The listing builds one solid part. Answer for the finished solid, in the listing's coordinates (mm). A direction names the side the tool comes from. Round coordinates to 2 decimals unless told otherwise and drop trailing zeros. Loops run counter-clockwise (first coordinate to the right, second up) from the corner with the lowest first, then second, coordinate; pieces in that order, holes last. Notation, with made-up numbers: M 8.5,-38 L 43.5,-38 A10 ccw 43.5,-20 Z; hole C 34.5,64 d11. An arc over 180 degrees is marked long. Answer as a JSON object with one key per item and string values.
```python
from build123d import *

# Parameters (mm, degrees)
F1_DEPTH = 20
F2_R     = 2
F3_R     = 3.25
F4_DEPTH = 50
F5_R     = 3.25
F6_DEPTH = 25


with BuildPart() as f1:
    # F0 (on Top) → F1 (new body)
    with BuildSketch(Plane.XY):
        with BuildLine():
            Line((0, 32), (0, 0))
            Line((0, 0), (1.5, 0))
            Line((1.5, 0), (1.5, 32))
            ThreePointArc((1.5, 32), (1.93934, 33.06066), (3, 33.5))
            Line((3, 33.5), (15, 33.5))
            ThreePointArc((15, 33.5), (17.12132, 34.37868), (18, 36.5))
            Line((18, 36.5), (18, 50))
            Line((18, 50), (16.5, 50))
            Line((16.5, 50), (16.5, 36.5))
            ThreePointArc((16.5, 36.5), (16.06066, 35.43934), (15, 35))
            Line((15, 35), (3, 35))
            ThreePointArc((3, 35), (0.87868, 34.12132), (0, 32))
        make_face()
    extrude(amount=F1_DEPTH)

    # F2
    f2_edges = [f1.edges().sort_by_distance(p)[0] for p in [
        (0.75, 0, 20),
        (0.75, 0, 0),
        (17.25, 50, 20),
        (17.25, 50, 0),
    ]]
    fillet(f2_edges, radius=F2_R)

    # F3 (on face) → F4 (cut)
    with BuildSketch(Plane.YZ.offset(18)):
        with Locations((9, 10)):
            Circle(F3_R)
    extrude(amount=-F4_DEPTH, mode=Mode.SUBTRACT)

    # F5 (on face) → F6 (cut)
    with BuildSketch(Plane.XZ.offset(-33.5)):
        with Locations((9, 10)):
            Circle(F5_R)
    extrude(amount=-F6_DEPTH, mode=Mode.SUBTRACT)


solid = f1.part
```
Item 1: The part is cut by section B-B (z = 10). Give the vertices of the cut face in (x, y).
Values follow:
{"outline": "M 0,0 L 1.5,0 L 1.5,5.75 L 0,5.75 Z; M 0,12.25 L 1.5,12.25 L 1.5,32 A1.5 cw 3,33.5 L 5.75,33.5 L 5.75,35 L 3,35 A3 ccw 0,32 Z; M 12.25,33.5 L 15,33.5 A3 ccw 18,36.5 L 18,50 L 16.5,50 L 16.5,36.5 A1.5 cw 15,35 L 12.25,35 Z"}
Item 2: Straight lines are drawn through the part: line 1 (Z direction, x = 0.4, y = 9); line 2 (Y direction, x = 7, z = 19); line 3 (X direction, y = 18, z = 1.5). For each, find the intervals that lie inside material, in ascending order.
Values follow:
{"line 1": "0 to 6.75, 13.25 to 20", "line 2": "33.5 to 35", "line 3": "0 to 1.5"}
Item 3: Flat-ended cylindrical pins translate along their axes: P1, Ø6, axis at y = 19, z = 8, coming from the +X side; P2, Ø2, axis at x = 15, z = 10, coming from the -Y side; P3, Ø6, axis at x = 6, z = 13.5, coming from the +Y side. Find the tip coordinate at first contact, or state that the pin passes through.
Values follow:
{"P1": "x = 1.5", "P2": "y = 33.5", "P3": "y = 35"}
Item 4: The part is cut by section C-C (y = 9). Give the vertices of the cut face in (x, z), then the cut area to 4 significant figures.
Values follow:
{"outline": "M 0,0 L 1.5,0 L 1.5,6.75 L 0,6.75 Z; M 0,13.25 L 1.5,13.25 L 1.5,20 L 0,20 Z", "area": "20.25 mm^2"}
Item 5: Determine the mould class of faces 4 (the face through (0.76, 0.57, 0.6)), 5 (the face through (16.5, 43, 10)), 6 (the face through (5.753, 34.24, 10.143)) for opening direction Z: released by +Z, released by -Z, zero draft, split by the parting line, or undercut.
Values follow:
{"face 4": "released by -Z", "face 5": "zero draft", "face 6": "undercut"}
Item 6: The part is cut by section A-A (x = 9). Give the vertices of the cut face in (y, z), then the cut area to 4 significant figures.
Values follow:
{"outline": "M 33.5,0 L 35,0 L 35,6.75 L 33.5,6.75 Z; M 33.5,13.25 L 35,13.25 L 35,20 L 33.5,20 Z", "area": "20.25 mm^2"}
Item 7: Which of the six approach directions +Z, -Z, +X, -X, +Y, -Y give full straight-line access (tool end or side, diameter ignored) to faces 1 (the face through (1.5, 16, 10)), 2 (the face through (6, 35, 8)), 3 (the face through (1, 27, 20))?
Values follow:
{"face 1": "+Z, -Z, +X, -Y", "face 2": "+Z, -Z, -X, +Y", "face 3": "+Z, +X, -X, +Y, -Y"}
Item 8: The part is cut by section D-D (z = 5.75). Give the vertices of the cut face in (x, y), then the cut area to 3 significant figures.
Values follow:
{"outline": "M 0,0 L 1.5,0 L 1.5,32 A1.5 cw 3,33.5 L 15,33.5 A3 ccw 18,36.5 L 18,50 L 16.5,50 L 16.5,36.5 A1.5 cw 15,35 L 3,35 A3 ccw 0,32 Z", "area": "96.9 mm^2"}
